```python
from build123d import *

# Parameters (mm, degrees)
BOSS_EXTRUDE1_DEPTH = 330.2
CUT_EXTRUDE1_REACH  = 27.4
SKETCH2_R           = 12.7
SKETCH3_R           = 2.667
CUT_EXTRUDE2_DEPTH  = 51.8
CUT_EXTRUDE3_REACH  = 27.4
SKETCH4_R           = 2.5908
CUT_EXTRUDE4_REACH  = 27.4
CUT_EXTRUDE5_DEPTH  = 51.8
CUT_EXTRUDE6_DEPTH  = 26.4


with BuildPart() as part:
    # Sketch1 → Boss-Extrude1 (new body)
    with BuildSketch(Plane.XY):
        Polygon((47.625, 3.175), (47.625, 25.4), (50.8, 25.4), (50.8, 0), (0, 0), (0, 25.4), (3.175, 25.4), (3.175, 3.175), align=None)
    extrude(amount=BOSS_EXTRUDE1_DEPTH)

    # Sketch2 → Cut-Extrude1 (cut, up to next)
    with BuildSketch(Plane.XZ, mode=Mode.PRIVATE) as cut_extrude1_sk1:
        with Locations((25.4, 298.45)):
            Circle(SKETCH2_R)
    cut_extrude1_tool1 = extrude(cut_extrude1_sk1.sketch, amount=-CUT_EXTRUDE1_REACH, mode=Mode.PRIVATE) & part.part
    add(cut_extrude1_tool1.solids().sort_by_distance((25.4, 0, 298.45))[0], mode=Mode.SUBTRACT)

    # Sketch3 → Cut-Extrude2 (cut, through all)
    with BuildSketch(Plane(origin=(50.8, 0, 0), x_dir=(0, 0, -1), z_dir=(1, 0, 0))):
        with Locations((-12.7, 12.7)):
            Circle(SKETCH3_R)
        with Locations((-50.8, 12.7)):
            Circle(SKETCH3_R)
    extrude(amount=-CUT_EXTRUDE2_DEPTH, mode=Mode.SUBTRACT)

    # Sketch4 → Cut-Extrude3 (cut, up to next)
    with BuildSketch(Plane.XZ, mode=Mode.PRIVATE) as cut_extrude3_sk1:
        with Locations((13.49375, 277.827770072)):
            Circle(SKETCH4_R)
    cut_extrude3_tool1 = extrude(cut_extrude3_sk1.sketch, amount=-CUT_EXTRUDE3_REACH, mode=Mode.PRIVATE) & part.part
    add(cut_extrude3_tool1.solids().sort_by_distance((13.49375, 0, 277.82777))[0], mode=Mode.SUBTRACT)
    # Sketch4 → Cut-Extrude3 (cut, up to next)
    with BuildSketch(Plane.XZ, mode=Mode.PRIVATE) as cut_extrude3_sk2:
        with Locations((37.30625, 277.827770072)):
            Circle(SKETCH4_R)
    cut_extrude3_tool2 = extrude(cut_extrude3_sk2.sketch, amount=-CUT_EXTRUDE3_REACH, mode=Mode.PRIVATE) & part.part
    add(cut_extrude3_tool2.solids().sort_by_distance((37.30625, 0, 277.82777))[0], mode=Mode.SUBTRACT)
    # Sketch4 → Cut-Extrude3 (cut, up to next)
    with BuildSketch(Plane.XZ, mode=Mode.PRIVATE) as cut_extrude3_sk3:
        with Locations((13.49375, 319.072229928)):
            Circle(SKETCH4_R)
    cut_extrude3_tool3 = extrude(cut_extrude3_sk3.sketch, amount=-CUT_EXTRUDE3_REACH, mode=Mode.PRIVATE) & part.part
    add(cut_extrude3_tool3.solids().sort_by_distance((13.49375, 0, 319.07223))[0], mode=Mode.SUBTRACT)
    # Sketch4 → Cut-Extrude3 (cut, up to next)
    with BuildSketch(Plane.XZ, mode=Mode.PRIVATE) as cut_extrude3_sk4:
        with Locations((37.30625, 319.072229928)):
            Circle(SKETCH4_R)
    cut_extrude3_tool4 = extrude(cut_extrude3_sk4.sketch, amount=-CUT_EXTRUDE3_REACH, mode=Mode.PRIVATE) & part.part
    add(cut_extrude3_tool4.solids().sort_by_distance((37.30625, 0, 319.07223))[0], mode=Mode.SUBTRACT)

    # Sketch5 → Cut-Extrude4 (cut, up to next)
    with BuildSketch(Plane.XZ, mode=Mode.PRIVATE) as cut_extrude4_sk1:
        with BuildLine():
            Line((40.122328379, 85.773383183), (15.196310059, 44.230019316))
            ThreePointArc((15.196310059, 44.230019316), (9.841228816, 42.090613006), (6.35, 46.680305352))
            Line((6.35, 46.680305352), (6.35, 88.223669219))
            ThreePointArc((6.35, 88.223669219), (7.744903955, 91.591265264), (11.1125, 92.986169219))
            Line((11.1125, 92.986169219), (36.03851832, 92.986169219))
            ThreePointArc((36.03851832, 92.986169219), (40.182845376, 90.570147325), (40.122328379, 85.773383183))
        make_face()
    cut_extrude4_tool1 = extrude(cut_extrude4_sk1.sketch, amount=-CUT_EXTRUDE4_REACH, mode=Mode.PRIVATE) & part.part
    add(cut_extrude4_tool1.solids().sort_by_distance((19.256233, 0, 73.00095))[0], mode=Mode.SUBTRACT)
    # Sketch5 → Cut-Extrude4 (cut, up to next)
    with BuildSketch(Plane.XZ, mode=Mode.PRIVATE) as cut_extrude4_sk2:
        with BuildLine():
            Line((14.76148168, 17.143987708), (39.6875, 17.143987708))
            ThreePointArc((39.6875, 17.143987708), (43.055096045, 18.538891662), (44.45, 21.906487708))
            Line((44.45, 21.906487708), (44.45, 63.449851575))
            ThreePointArc((44.45, 63.449851575), (40.958771184, 68.03954392), (35.603689941, 65.90013761))
            Line((35.603689941, 65.90013761), (10.677671621, 24.356773743))
            ThreePointArc((10.677671621, 24.356773743), (10.617154624, 19.560009601), (14.76148168, 17.143987708))
        make_face()
    cut_extrude4_tool2 = extrude(cut_extrude4_sk2.sketch, amount=-CUT_EXTRUDE4_REACH, mode=Mode.PRIVATE) & part.part
    add(cut_extrude4_tool2.solids().sort_by_distance((31.543767, 0, 37.129207))[0], mode=Mode.SUBTRACT)
    # Sketch5 → Cut-Extrude4 (cut, up to next)
    with BuildSketch(Plane.XZ, mode=Mode.PRIVATE) as cut_extrude4_sk3:
        with BuildLine():
            Line((40.122328379, 167.965564694), (15.196310059, 126.422200827))
            ThreePointArc((15.196310059, 126.422200827), (9.841228816, 124.282794517), (6.35, 128.872486862))
            Line((6.35, 128.872486862), (6.35, 170.415850729))
            ThreePointArc((6.35, 170.415850729), (7.744903955, 173.783446775), (11.1125, 175.178350729))
            Line((11.1125, 175.178350729), (36.03851832, 175.178350729))
            ThreePointArc((36.03851832, 175.178350729), (40.182845376, 172.762328836), (40.122328379, 167.965564694))
        make_face()
    cut_extrude4_tool3 = extrude(cut_extrude4_sk3.sketch, amount=-CUT_EXTRUDE4_REACH, mode=Mode.PRIVATE) & part.part
    add(cut_extrude4_tool3.solids().sort_by_distance((19.256233, 0, 155.193132))[0], mode=Mode.SUBTRACT)
    # Sketch5 → Cut-Extrude4 (cut, up to next)
    with BuildSketch(Plane.XZ, mode=Mode.PRIVATE) as cut_extrude4_sk4:
        with BuildLine():
            Line((14.76148168, 99.336169219), (39.6875, 99.336169219))
            ThreePointArc((39.6875, 99.336169219), (43.055096045, 100.731073173), (44.45, 104.098669219))
            Line((44.45, 104.098669219), (44.45, 145.642033085))
            ThreePointArc((44.45, 145.642033085), (40.958771184, 150.231725431), (35.603689941, 148.092319121))
            Line((35.603689941, 148.092319121), (10.677671621, 106.548955254))
            ThreePointArc((10.677671621, 106.548955254), (10.617154624, 101.752191112), (14.76148168, 99.336169219))
        make_face()
    cut_extrude4_tool4 = extrude(cut_extrude4_sk4.sketch, amount=-CUT_EXTRUDE4_REACH, mode=Mode.PRIVATE) & part.part
    add(cut_extrude4_tool4.solids().sort_by_distance((31.543767, 0, 119.321388))[0], mode=Mode.SUBTRACT)
    # Sketch5 → Cut-Extrude4 (cut, up to next)
    with BuildSketch(Plane.XZ, mode=Mode.PRIVATE) as cut_extrude4_sk5:
        with BuildLine():
            Line((40.122328379, 250.157746205), (15.196310059, 208.614382338))
            ThreePointArc((15.196310059, 208.614382338), (9.841228816, 206.474976028), (6.35, 211.064668373))
            Line((6.35, 211.064668373), (6.35, 252.60803224))
            ThreePointArc((6.35, 252.60803224), (7.744903955, 255.975628285), (11.1125, 257.37053224))
            Line((11.1125, 257.37053224), (36.03851832, 257.37053224))
            ThreePointArc((36.03851832, 257.37053224), (40.182845376, 254.954510346), (40.122328379, 250.157746205))
        make_face()
    cut_extrude4_tool5 = extrude(cut_extrude4_sk5.sketch, amount=-CUT_EXTRUDE4_REACH, mode=Mode.PRIVATE) & part.part
    add(cut_extrude4_tool5.solids().sort_by_distance((19.256233, 0, 237.385313))[0], mode=Mode.SUBTRACT)
    # Sketch5 → Cut-Extrude4 (cut, up to next)
    with BuildSketch(Plane.XZ, mode=Mode.PRIVATE) as cut_extrude4_sk6:
        with BuildLine():
            Line((14.76148168, 181.528350729), (39.6875, 181.528350729))
            ThreePointArc((39.6875, 181.528350729), (43.055096045, 182.923254684), (44.45, 186.290850729))
            Line((44.45, 186.290850729), (44.45, 227.834214596))
            ThreePointArc((44.45, 227.834214596), (40.958771184, 232.423906942), (35.603689941, 230.284500631))
            Line((35.603689941, 230.284500631), (10.677671621, 188.741136765))
            ThreePointArc((10.677671621, 188.741136765), (10.617154624, 183.944372623), (14.76148168, 181.528350729))
        make_face()
    cut_extrude4_tool6 = extrude(cut_extrude4_sk6.sketch, amount=-CUT_EXTRUDE4_REACH, mode=Mode.PRIVATE) & part.part
    add(cut_extrude4_tool6.solids().sort_by_distance((31.543767, 0, 201.51357))[0], mode=Mode.SUBTRACT)

    # Sketch6 → Cut-Extrude5 (cut, through all)
    with BuildSketch(Plane.ZY):
        with BuildLine():
            Line((78.616971835, 19.05), (129.416971835, 19.05))
            ThreePointArc((129.416971835, 19.05), (135.766971835, 12.7), (129.416971835, 6.35))
            Line((129.416971835, 6.35), (78.616971835, 6.35))
            ThreePointArc((78.616971835, 6.35), (72.266971835, 12.7), (78.616971835, 19.05))
        make_face()
        with BuildLine():
            Line((148.466971835, 19.05), (199.266971835, 19.05))
            ThreePointArc((199.266971835, 19.05), (205.616971835, 12.7), (199.266971835, 6.35))
            Line((199.266971835, 6.35), (148.466971835, 6.35))
            ThreePointArc((148.466971835, 6.35), (142.116971835, 12.7), (148.466971835, 19.05))
        make_face()
    extrude(amount=-CUT_EXTRUDE5_DEPTH, mode=Mode.SUBTRACT)

    # Sketch7 → Cut-Extrude6 (cut, through all)
    with BuildSketch(Plane.XZ):
        Polygon((0, 330.2), (0, 315.558408634), (14.641591366, 330.2), align=None)
        Polygon((36.158408634, 330.2), (50.8, 330.2), (50.8, 315.558408634), align=None)
    extrude(amount=-CUT_EXTRUDE6_DEPTH, mode=Mode.SUBTRACT)


solid = part.part
```
Geometry check sheet. Reference: the model listing, model coordinates, mm. A direction names the side the tool comes from. Round coordinates to 2 decimals unless told otherwise and drop trailing zeros. Order: outer loops, then holes, each group sorted by start corner. A loop starts at its lowest first (then second) coordinate and runs counter-clockwise, first axis right, second up. Notation, with made-up numbers: (44, -8.5) - (48, -8.5) arc R32 cw to (48, 19.5) - close; hole circle Ø1 at (14, 7.5). An arc over 180 degrees is marked (long way). Use a Markdown table: item, result. Add a question column.
1) Section check B-B (y = 22.5). Record the cut outline in (x, z) (3 decimals).
2) Set-up check for faces 5 (the flat face through (23.315, 1.565, 209.804)), 6 (the flat face through (2.95, 9.82, 318.51)), 7 (the flat face through (3.175, 19.4, 157.1)), 8 (the cylindrical face through (49.19, 12.84, 205.615)): record each of +Z, -Z, +X, -X, +Y, -Y from which the full face is reachable in a straight line by a thin tool's end or side.
3) Mould release check, pull along X, two halves, no side actions. Record for faces 1 (the flat face through (0, 21, 156)), 2 (the flat face through (47.85, 9.82, 318.51)), 3 (the flat face through (40, 3.175, 163)), 4 (the cylindrical face through (1.61, 12.817, 53.464)): released by +X, released by -X, zero draft, split by the parting line, or undercut.
4) Gauge pin test, flat ends, axial feed: P1, Ø4.5, axis at y = 12.7, z = 50.8, coming from the +X side; P2, Ø4, axis at x = 26.5, z = 94.5, coming from the -Y side. Record the tip position at first contact, or that the pin passes through.
5) Section check A-A (z = 298.45). Record the cut outline in (x, y) (3 decimals), then the cut area to 3 significant figures.
6) Section check D-D (z = 118). Record the cut outline in (x, y) (3 decimals).
7) Thickness scan on line 1 along X through (y, z) = (22.5, 174) (3 decimals); line 2 along Y through (x, z) = (2, 81); line 3 along Y through (x, z) = (46, 39) (3 decimals). Record the ranges inside material, lowest first.
8) Section check C-C (x = 25.4). Count the separate pieces of the cut face and the enclosed holes in it, then the cut area to 3 significant figures.
Established:
| question | item | result |
|---|---|---|
| 1 | outline | (0, 0) - (3.175, 0) - (3.175, 318.733) - (0, 315.558) - close; (47.625, 0) - (50.8, 0) - (50.8, 315.558) - (47.625, 318.733) - close |
| 2 | face 5 | +Y, -Y |
| 2 | face 6 | +Z, -X, +Y, -Y |
| 2 | face 7 | +Z, -Z, +Y |
| 2 | face 8 | +X, -X |
| 3 | face 1 | released by -X |
| 3 | face 2 | released by +X |
| 3 | face 3 | undercut |
| 3 | face 4 | zero draft |
| 4 | P1 | through |
| 4 | P2 | y = 0 |
| 5 | outline | (0, 0) - (12.7, 0) - (12.7, 3.175) - (3.175, 3.175) - (3.175, 25.4) - (0, 25.4) - close; (38.1, 0) - (50.8, 0) - (50.8, 25.4) - (47.625, 25.4) - (47.625, 3.175) - (38.1, 3.175) - close |
| 5 | area | 222 mm2 |
| 6 | outline | (0, 0) - (17.548, 0) - (17.548, 3.175) - (3.175, 3.175) - (3.175, 6.35) - (0, 6.35) - close; (0, 19.05) - (3.175, 19.05) - (3.175, 25.4) - (0, 25.4) - close; (44.45, 0) - (50.8, 0) - (50.8, 6.35) - (47.625, 6.35) - (47.625, 3.175) - (44.45, 3.175) - close; (47.625, 19.05) - (50.8, 19.05) - (50.8, 25.4) - (47.625, 25.4) - close |
| 7 | line 1 | 0 to 3.175, 47.625 to 50.8 |
| 7 | line 2 | 0 to 6.35, 19.05 to 25.4 |
| 7 | line 3 | 0 to 3.175 |
| 8 | separate pieces | 8 |
| 8 | enclosed holes | 0 |
| 8 | area | 363 mm2 |
